Geometry check sheet. Reference: the model listing, model coordinates, mm. A direction names the side the tool comes from. Coordinates: 2 decimals unless noted, no trailing zeros. Answer in a Markdown table with one row per item. Add a question column.
Q1. Gauge pin test, flat ends, axial feed: P1, Ø3.5, axis at x = 86.5, y = -78, coming from the +Z side; P2, Ø4.5, axis at x = 90.41, y = 77.08, coming from the -Z side. Record the tip position at first contact, or that the pin passes through.
Q2. Tool access check on faces 1 (the face through (-2, -86.548, 5)), 2 (the face through (86.27, 81.59, 8.19)). Record the directions out of +Z, -Z, +X, -X, +Y, -Y that give a thin tool (end or side, any length) a straight path to the whole face; none if there is none.
Q3. Thickness scan on line 1 (X direction, y = -77, z = 4.25); line 2 (Y direction, x = -108, z = 8.75); line 3 (X direction, y = 79, z = 6.5). Record the ranges inside material, lowest first.
Q4. Release check for a two-part mould opening along X. For faces 3 (the face through (-2, 103.452, 5)), 4 (the face through (-125, 7, 5)), 5 (the face through (125, 7, 5)), 6 (the face through (85.42, -76.62, 3.22)) record: pulls with the +X half, pulls with the -X half, needs draft (parallel to the pull), parting line crosses it, or undercut.
```python
from build123d import *

# Parameters (mm, degrees)
SKETCH1_W                                   = 250
SKETCH1_H                                   = 190
BOSS_EXTRUDE1_DEPTH                         = 10
CBORE_FOR_M5_HEX_HEAD_CAP_SCREW1_AT_2_COUNT = 2
CBORE_FOR_M5_HEX_HEAD_CAP_SCREW1_AT_2_PITCH = 174.025024549
CBORE_FOR_M5_HEX_HEAD_CAP_SCREW1_AT_3_COUNT = 2
CBORE_FOR_M5_HEX_HEAD_CAP_SCREW1_AT_3_PITCH = 261.850395634
CBORE_FOR_M5_HEX_HEAD_CAP_SCREW1_AT_4_COUNT = 2
CBORE_FOR_M5_HEX_HEAD_CAP_SCREW1_AT_4_PITCH = 200


with BuildPart() as part:
    # Sketch1 → Boss-Extrude1 (new body)
    with BuildSketch(Plane.XY):
        with Locations((0, 8.452072107)):
            Rectangle(SKETCH1_W, SKETCH1_H)
    extrude(amount=BOSS_EXTRUDE1_DEPTH)

    # Sketch10 → CBORE for M5 Hex Head Cap Screw1 (revolve, cut)
    with BuildSketch(Plane(origin=(-108.749145678, 95.452072107, 10), x_dir=(0, -1, 0), z_dir=(1, 0, 0))):
        Polygon((0, 0), (0, 10), (2.9, 10), (2.9, 3.65), (6.12, 3.65), (6.12, 0.025), (6.145, 0), align=None)
    cbore_for_m5_hex_head_cap_screw1 = revolve(axis=Axis((-108.749145678, 95.452072107, 16.35), (0, 0, -1)), mode=Mode.SUBTRACT)

    # CBORE for M5 Hex Head Cap Screw1 at 2: CBORE for M5 Hex Head Cap Screw1 ×2
    with Locations(*[Vector(-0.01695807915079003, -0.9998562014367444, 0) * (i * CBORE_FOR_M5_HEX_HEAD_CAP_SCREW1_AT_2_PITCH) for i in range(1, CBORE_FOR_M5_HEX_HEAD_CAP_SCREW1_AT_2_COUNT)]):
        add(cbore_for_m5_hex_head_cap_screw1, mode=Mode.SUBTRACT)

    # CBORE for M5 Hex Head Cap Screw1 at 3: CBORE for M5 Hex Head Cap Screw1 ×2
    with Locations(*[Vector(0.7525017460823102, -0.6585902536046783, 0) * (i * CBORE_FOR_M5_HEX_HEAD_CAP_SCREW1_AT_3_PITCH) for i in range(1, CBORE_FOR_M5_HEX_HEAD_CAP_SCREW1_AT_3_COUNT)]):
        add(cbore_for_m5_hex_head_cap_screw1, mode=Mode.SUBTRACT)

    # CBORE for M5 Hex Head Cap Screw1 at 4: CBORE for M5 Hex Head Cap Screw1 ×2
    with Locations(*[Vector(0.9957709917740633, -0.09187019071112518, 0) * (i * CBORE_FOR_M5_HEX_HEAD_CAP_SCREW1_AT_4_PITCH) for i in range(1, CBORE_FOR_M5_HEX_HEAD_CAP_SCREW1_AT_4_COUNT)]):
        add(cbore_for_m5_hex_head_cap_screw1, mode=Mode.SUBTRACT)


solid = part.part
```
Calculated:
| question | item | result |
|---|---|---|
| 1 | P1 | stops at z = 6.35 |
| 1 | P2 | passes through |
| 2 | face 1 | +Z, -Z, +X, -X, -Y |
| 2 | face 2 | +Z |
| 3 | line 1 | x = -125 to -114.15, -109.25 to 85.39, 91.19 to 125 |
| 3 | line 2 | y = -86.55 to -83.42, -73.67 to 89.38, 101.53 to 103.45 |
| 3 | line 3 | x = -125 to 84.59, 96.22 to 125 |
| 4 | face 3 | needs draft |
| 4 | face 4 | pulls with the -X half |
| 4 | face 5 | pulls with the +X half |
| 4 | face 6 | undercut |
